Geometry: final body of the model. Coordinates: model frame, mm. A direction names the side the tool comes from. Round coordinates to 2 decimals unless told otherwise and drop trailing zeros. Loops run counter-clockwise (first coordinate to the right, second up) from the corner with the lowest first, then second, coordinate; pieces in that order, holes last. Notation, with made-up numbers: (-24.5, -11.75) - (27.5, -11.75) arc R14 ccw to (27.5, 7.25) - close; hole circle Ø5 at (72, 18.5). An arc over 180 degrees is marked (long way). Answer in a Markdown table with one row per item. Add a question column.
Autodesk Fusion 360 part; units mm, degrees
sketch "Sketch1" plane through (0, 0, 0) normal (0, 1, 0) x (1, 0, 0)
  line L0 (0, 0) -> (12.5, 0)
  line L1 (12.5, 0) -> (12.5, 24)
  line L2 (12.5, 24) -> (0, 24)
  line L3 (0, 24) -> (0, 0)
  dimension "d1" = 12.5
  dimension "d2" = 24
extrude "Extrude1" add sketch "Sketch1" along normal blind 1.5
extrude "Extrude2" add 1 faces at (0, 0.5, -16) along direction (-1, 0, 0) blind 1.5
extrude "Extrude3" add 1 faces at (12.5, 0.5, -8) along direction (1, 0, 0) blind 1.5
sketch "Sketch2" plane through (0, 1.5, 0) normal (0, 1, 0) x (-1, 0, 0)
  line L0 (1.5, 0) -> (-14, 0)
  line L1 (-14, 0) -> (-14, -24)
  line L2 (-14, -24) -> (1.5, -24)
  line L3 (1.5, -24) -> (1.5, 0)
  line L4 (1.5, -24) -> (0, -24)
  line L5 (0, -24) -> (0, 0)
  line L6 (0, 0) -> (1.5, 0)
  line L7 (1.5, 0) -> (1.5, -24)
  line L8 (-14, -24) -> (-12.5, -24)
  line L9 (-12.5, -24) -> (-12.5, 0)
  line L10 (-12.5, 0) -> (-14, 0)
  line L11 (-14, 0) -> (-14, -24)
  dimension "d9" = 1.5
extrude "Extrude4" add sketch "Sketch2" along normal blind 10 contours L0 L2 L3 L4 L5 L6 L7 | L0 L1 L2 L8 L9 L10 L11
sketch "Sketch3" plane through (14, 0, 0) normal (1, 0, 0) x (0, 0, -1)
  line L0 (0, 0) -> (24, 0)
  line L1 (24, 0) -> (24, 11.5)
  line L2 (24, 11.5) -> (0, 11.5)
  line L3 (0, 11.5) -> (0, 0)
  line L4 (0, 11.5) -> (24, 11.5)
  line L5 (24, 11.5) -> (24, 10.5)
  line L6 (24, 10.5) -> (0, 10.5)
  line L7 (0, 10.5) -> (0, 11.5)
  dimension "d12" = 1
extrude "Extrude5" add sketch "Sketch3" along normal blind 5 contours L1 L2 L3 L4 L5 L6 L7
sketch "Sketch4" plane through (-1.5, 0, 0) normal (-1, 0, 0) x (0, 0, 1)
  line L0 (-24, 0) -> (0, 0)
  line L1 (0, 0) -> (0, 11.5)
  line L2 (0, 11.5) -> (-24, 11.5)
  line L3 (-24, 11.5) -> (-24, 0)
  line L4 (-24, 11.5) -> (0, 11.5)
  line L5 (0, 11.5) -> (0, 10.5)
  line L6 (0, 10.5) -> (-24, 10.5)
  line L7 (-24, 10.5) -> (-24, 11.5)
  dimension "d15" = 1
extrude "Extrude6" add sketch "Sketch4" along normal blind 5 contours L1 L2 L3 L4 L5 L6 L7
ref_plane "WorkPlane1" through (-4, 10.5, -12) normal (0, -1, 0) x (0, 0, 1)
sketch "Sketch5" plane through (-4, 10.5, -12) normal (0, -1, 0) x (1, 0, 0)
  line L0 (23, 12) -> (23, -12)
  line L1 (-2.5, -12) -> (-2.5, 12)
  point P0 (0.09, 9.9032)
  point P1 (20.41, 9.9032)
  point P2 (0.09, 7.3632)
  point P3 (0.09, 4.8232)
  point P4 (0.09, 2.2832)
  point P5 (0.09, -0.2568)
  point P6 (0.09, -2.7968)
  point P7 (0.09, -5.3368)
  point P8 (0.09, -7.8768)
  point P9 (0.09, -10.4168)
  point P10 (20.41, 7.3632)
  point P11 (20.41, 4.8232)
  point P12 (20.41, 2.2832)
  point P13 (20.41, -0.2568)
  point P14 (20.41, -2.7968)
  point P15 (20.41, -5.3368)
  point P16 (20.41, -7.8768)
  point P17 (20.41, -10.4168)
  dimension "d19" = 20.32
  dimension "d20" = 2.59
  dimension "d21" = 2.59
  dimension "d24" = 0
  dimension "d25" = -20.32
  dimension "d28" = 0
  dimension "d29" = -20.32
hole "Hole1" at (-3.91, 10.5, -2.0968) at (-3.91, 10.5, -4.6368) at (-3.91, 10.5, -7.1768) at (-3.91, 10.5, -9.7168) at (-3.91, 10.5, -12.2568) at (-3.91, 10.5, -14.7968) at (-3.91, 10.5, -17.3368) at (-3.91, 10.5, -19.8768) at (-3.91, 10.5, -22.4168) at (16.41, 10.5, -2.0968) at (16.41, 10.5, -4.6368) at (16.41, 10.5, -7.1768) at (16.41, 10.5, -9.7168) at (16.41, 10.5, -12.2568) at (16.41, 10.5, -14.7968) at (16.41, 10.5, -17.3368) at (16.41, 10.5, -19.8768) at (16.41, 10.5, -22.4168) direction (0, 1, 0) diameter 1 depth 7 tip angle 118
sketch "Sketch6" plane through (0, 1.5, 0) normal (0, 1, 0) x (-1, 0, 0)
  line L0 (-12.5, 0) -> (-12.5, -24)
  line L1 (-12.5, -24) -> (0, -24)
  line L2 (0, -24) -> (0, 0)
  line L3 (0, 0) -> (-12.5, 0)
  line L4 (0, -18) -> (-5, -18)
  line L5 (-5, -18) -> (-5, -16)
  line L6 (-5, -16) -> (0, -16)
  line L7 (0, -16) -> (0, -18)
  dimension "d33" = 5
  dimension "d34" = 2
  dimension "d35" = 6
extrude "Extrude7" add sketch "Sketch6" along normal blind 2 contours L2 L4 L5 L6 L7
fillet "Fillet1" radius 1 2 edges at (-1.5, 0, -12) (14, 0, -12)
fillet "Fillet2" radius 0.5 2 edges at (0, 11.5, -12) (12.5, 11.5, -12)
fillet "Fillet3" radius 1.5 4 edges at (19, 11, -24) (19, 11, 0) (-6.5, 11, 0) (-6.5, 11, -24)
fillet "Fillet4" radius 0.5 3 edges at (5, 3.5, -17) (2.5, 3.5, -18) (2.5, 3.5, -16)
1) Section A-A, the plane y = 9.5. Return the cut outline in (x, z).
2) Reachability of faces 4 (the flat face through (3, 2, -16)), 5 (the flat face through (2, 2, -18)), 6 (the flat face through (12.5, 6, -12)) from +Z, -Z, +X, -X, +Y, -Y: full face, straight path, thin tool, end or side. Return the list, or none.
3) Section B-B, the plane z = -13.75. Return the cut outline in (x, y).
4) Pull-direction query (X, two-part tool) for faces 1 (the flat face through (18, 10.5, -12)), 2 (the cylindrical face through (-3.932, 11.007, -14.297)), 3 (the cylindrical face through (13.715, 0.301, -12.168)); classes: pulls with the +X half, pulls with the -X half, needs draft (parallel to the pull), parting line crosses it, or undercut.
5) Section C-C, the plane x = 16.41. Give the number of separate pieces and of enclosed holes in the cut face, and give its area (3 significant figures).
6) Section D-D, the plane z = -20. Return the cut outline in (x, y).
7) Material intervals for line 1 along X through (y, z) = (6.75, -21.75); line 2 along X through (y, z) = (11, -4.75); line 3 along Y through (x, z) = (-3.5, -22.75), sorted ascending. Write a range as from..to.
8) Contact query for flat-ended pins moving along their axis: pin 1 Ø1 at (x, z) = (15.5, -9.5) entering from -Y; pin 2 Ø6 at (x, z) = (6.5, -18) entering from +Y; pin 3 Ø5 at (y, z) = (5, -12.5) entering from -X. Output: stop coordinate, or through.
Evaluation:
| question | item | result |
|---|---|---|
| 1 | outline | (-1.5, -24) - (0, -24) - (0, 0) - (-1.5, 0) - close; (12.5, -24) - (14, -24) - (14, 0) - (12.5, 0) - close |
| 2 | face 4 | +Z, +Y |
| 2 | face 5 | -Z, +Y |
| 2 | face 6 | +Z, -Z, +Y |
| 3 | outline | (-6.5, 10.5) - (-1.5, 10.5) - (-1.5, 1) arc R1 ccw to (-0.5, 0) - (13, 0) arc R1 ccw to (14, 1) - (14, 10.5) - (19, 10.5) - (19, 11.5) - (13, 11.5) arc R0.5 ccw to (12.5, 11) - (12.5, 1.5) - (0, 1.5) - (0, 11) arc R0.5 ccw to (-0.5, 11.5) - (-6.5, 11.5) - close |
| 4 | face 1 | needs draft |
| 4 | face 2 | undercut |
| 4 | face 3 | pulls with the +X half |
| 5 | separate pieces | 10 |
| 5 | enclosed holes | 0 |
| 5 | area | 15.0 mm² |
| 6 | outline | (-6.5, 10.5) - (-4.39, 10.5) - (-4.39, 11.5) - (-6.5, 11.5) - close; (-3.43, 10.5) - (-1.5, 10.5) - (-1.5, 1) arc R1 ccw to (-0.5, 0) - (13, 0) arc R1 ccw to (14, 1) - (14, 10.5) - (15.93, 10.5) - (15.93, 11.5) - (13, 11.5) arc R0.5 ccw to (12.5, 11) - (12.5, 1.5) - (0, 1.5) - (0, 11) arc R0.5 ccw to (-0.5, 11.5) - (-3.43, 11.5) - close; (16.89, 10.5) - (19, 10.5) - (19, 11.5) - (16.89, 11.5) - close |
| 7 | line 1 | x = -1.5..0, 12.5..14 |
| 7 | line 2 | x = -6.5..-4.4, -3.42..0, 12.5..15.92, 16.9..19 |
| 7 | line 3 | y = 10.5..11.5 |
| 8 | pin 1 | stops at y = 10.5 |
| 8 | pin 2 | stops at y = 3.5 |
| 8 | pin 3 | stops at x = -1.5 |
